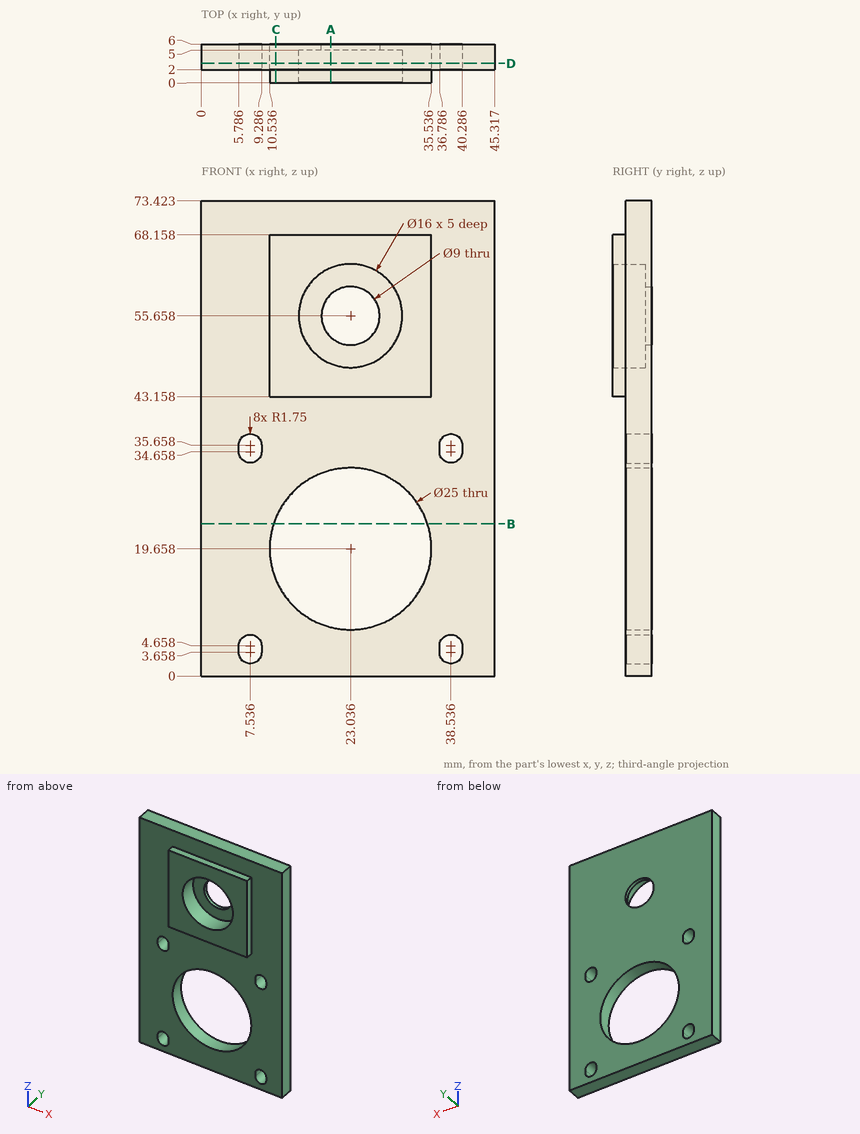
Can you work these out from the drawing? Everything is in mm from the part's minimum corner. Round coordinates to 2 decimals unless told otherwise and drop trailing zeros. Loops run counter-clockwise (first coordinate to the right, second up) from the corner with the lowest first, then second, coordinate; pieces in that order, holes last. Notation, with made-up numbers: (44, 3.5) -> (72, 3.5) arc R23 ccw to (72, 17.5) -> close; hole circle Ø10 at (7, 65). An arc over 180 degrees is marked (long way). Put each result on its own line as item: value.
Q1. I want a section at D-D on y = 3. Write out the boundary of the cut face in (x, z), and give its area (3 significant figures).
Checks:
outline: (0, 0) -> (45.32, 0) -> (45.32, 73.42) -> (0, 73.42) -> close; hole (5.79, 3.66) arc R1.75 ccw to (9.29, 3.66) -> (9.29, 4.66) arc R1.75 ccw to (5.79, 4.66) -> close; hole (5.79, 34.66) arc R1.75 ccw to (9.29, 34.66) -> (9.29, 35.66) arc R1.75 ccw to (5.79, 35.66) -> close; hole circle Ø25 at (23.04, 19.66); hole circle Ø16 at (23.04, 55.66); hole (36.79, 3.66) arc R1.75 ccw to (40.29, 3.66) -> (40.29, 4.66) arc R1.75 ccw to (36.79, 4.66) -> close; hole (36.79, 34.66) arc R1.75 ccw to (40.29, 34.66) -> (40.29, 35.66) arc R1.75 ccw to (36.79, 35.66) -> close
area: 2,580 mm2
Q2. I want a section at A-A on x = 20. Write out the boundary of the cut face in (y, z).
Checks:
outline: (0, 43.16) -> (2, 43.16) -> (2, 31.78) -> (6, 31.78) -> (6, 52.34) -> (5, 52.34) -> (5, 48.26) -> (0, 48.26) -> close; (0, 63.06) -> (5, 63.06) -> (5, 58.98) -> (6, 58.98) -> (6, 73.42) -> (2, 73.42) -> (2, 68.16) -> (0, 68.16) -> close; (2, 0) -> (6, 0) -> (6, 7.53) -> (2, 7.53) -> close
Q3. I want a section at C-C on x = 11.5. Write out the boundary of the cut face in (y, z) (1 decimal), and give its area (3 significant figures).
Checks:
outline: (0, 43.2) -> (2, 43.2) -> (2, 24.5) -> (6, 24.5) -> (6, 73.4) -> (2, 73.4) -> (2, 68.2) -> (0, 68.2) -> close; (2, 0) -> (6, 0) -> (6, 14.8) -> (2, 14.8) -> close
area: 305 mm2
Q4. Please list where these lines run through material, in increasing order: line 1 (X direction, y = 2.75, z = 20); line 2 (Z direction, x = 27.5, y = 2.15) (1 decimal); line 3 (Z direction, x = 8, y = 2.1) (1 decimal). Write a range as from..to.
Checks:
line 1: 0..10.54, 35.53..45.32
line 2: 0..8, 31.3..49, 62.3..73.4
line 3: 0..2, 6.3..33, 37.3..73.4
Q5. I want a section at B-B on z = 23.5. Write out the boundary of the cut face in (x, y), and give its area (3 significant figures).
Checks:
outline: (0, 2) -> (11.14, 2) -> (11.14, 6) -> (0, 6) -> close; (34.93, 2) -> (45.32, 2) -> (45.32, 6) -> (34.93, 6) -> close
area: 86.1 mm2
Q6. For pin 1 Ø1.5 at (x, z) = (27.5, 39) entering from -Y; pin 2 Ø1.6 at (x, y) = (22.5, 1) entering from +Z, each with a flat end and sliding along its axis, tell me the tip position at first contact or that it passes through.
Checks:
pin 1: y = 2
pin 2: z = 68.16
